from build123d import *

# Parameters (mm, degrees)
SKETCH1_W           = 7
SKETCH1_H           = 7
BOSS_EXTRUDE1_DEPTH = 3
CUT_EXTRUDE1_DEPTH  = 7
CUT_EXTRUDE2_DEPTH  = 11
SKETCH4_R           = 1.8
CUT_EXTRUDE3_DEPTH  = 0.8
CUT_EXTRUDE4_DEPTH  = 0.4


with BuildPart() as part:
    # Sketch1 → Boss-Extrude1 (new body)
    with BuildSketch(Plane(origin=(0, 0, 0), x_dir=(1, 0, 0), z_dir=(0, 1, 0))):
        with Locations((3.5, 3.5)):
            Rectangle(SKETCH1_W, SKETCH1_H)
    extrude(amount=BOSS_EXTRUDE1_DEPTH)

    # Sketch2 → Cut-Extrude1 (cut)
    with BuildSketch(Plane.XY):
        Polygon((0, 0), (0.7, 3), (0, 3), align=None)
        Polygon((7, 0), (6.3, 3), (7, 3), align=None)
    extrude(amount=-CUT_EXTRUDE1_DEPTH, mode=Mode.SUBTRACT)

    # Sketch3 → Cut-Extrude2 (cut)
    with BuildSketch(Plane(origin=(0, 0, 0), x_dir=(0, 0, -1), z_dir=(1, 0, 0))):
        Polygon((0, 0), (0.7, 3), (0, 3), align=None)
        Polygon((7, 3), (6.3, 3), (7, 0), align=None)
    extrude(amount=CUT_EXTRUDE2_DEPTH, mode=Mode.SUBTRACT)

    # Sketch4 → Cut-Extrude3 (cut)
    with BuildSketch(Plane.XZ):
        with Locations(Location((3.5, -3.5, 0), (0, 0, 270))):
            Circle(SKETCH4_R)
    extrude(amount=-CUT_EXTRUDE3_DEPTH, mode=Mode.SUBTRACT)

    # Sketch5 → Cut-Extrude4 (cut)
    with BuildSketch(Plane(origin=(0, 3, 0), x_dir=(1, 0, 0), z_dir=(0, 1, 0))):
        with BuildLine():
            Line((2.030546131, 1.772776287), (2.030546131, 5.272776287))
            Line((2.030546131, 5.272776287), (3.499396292, 5.272776287))
            add(Edge.make_bspline(
                [(3.499396292, 5.272776287), (3.5440361, 5.272501173), (3.63006518, 5.271970977), (3.754480014, 5.268104688), (3.869218418, 5.260004585), (3.974789374, 5.250831153), (4.070685816, 5.2374844), (4.157286901, 5.221495121), (4.23444683, 5.202965752), (4.303291413, 5.180773827), (4.366063686, 5.155374398), (4.424539139, 5.125141932), (4.479360726, 5.089720882), (4.531370453, 5.050332114), (4.580788559, 5.006915106), (4.626260263, 4.958320831), (4.668577803, 4.90527287), (4.707707034, 4.848212589), (4.742177437, 4.787391941), (4.773674335, 4.724764195), (4.799313998, 4.659662899), (4.820492127, 4.592394727), (4.837409543, 4.523105729), (4.849151659, 4.451619746), (4.856482135, 4.378066169), (4.857136528, 4.328382861), (4.857469208, 4.303124845)],
                knots=[0, 0, 0, 0, 1.675828044, 3.229627355, 4.67171229, 5.993455049, 7.206927059, 8.304770529, 9.29850117, 10.183580433, 11.017754134, 11.837875825, 12.650738409, 13.464925643, 14.285328857, 15.117007378, 15.959673368, 16.830859064, 17.711229498, 18.58228265, 19.460420693, 20.334473227, 21.228207035, 22.135446768, 23.052097822, 24, 24, 24, 24], degree=3))
            add(Edge.make_bspline(
                [(4.857469208, 4.303124845), (4.856852136, 4.271306813), (4.855646207, 4.20912561), (4.844548611, 4.117987318), (4.828065847, 4.030911185), (4.804569794, 3.947776576), (4.772263199, 3.869561272), (4.734759192, 3.795169587), (4.690029362, 3.724853862), (4.638377601, 3.659311167), (4.579850151, 3.598483484), (4.51419052, 3.543622601), (4.441867499, 3.494514108), (4.362443578, 3.451441194), (4.276471789, 3.414618521), (4.18357933, 3.383637045), (4.084186726, 3.358421575), (4.015049286, 3.346556943), (3.979664721, 3.34048462)],
                knots=[0, 0, 0, 0, 1.05911256, 2.069797862, 3.05271628, 4.008392045, 4.940519534, 5.866323021, 6.779546087, 7.71056835, 8.640711998, 9.585328432, 10.554502533, 11.547017206, 12.589327225, 13.664782803, 14.804835066, 16, 16, 16, 16], degree=3))
            add(Edge.make_bspline(
                [(3.979664721, 3.34048462), (4.013885569, 3.317819831), (4.080860431, 3.27346175), (4.173524973, 3.200403435), (4.256715746, 3.123723082), (4.319703603, 3.055534143), (4.368103279, 2.995569296), (4.407073288, 2.943123463), (4.44910869, 2.882765916), (4.493797209, 2.814463953), (4.542459952, 2.738821883), (4.593287063, 2.65468189), (4.647342172, 2.562864685), (4.683685664, 2.49872572), (4.702521292, 2.46548462)],
                knots=[0, 0, 0, 0, 1.285445069, 2.515791127, 3.691898215, 4.826622834, 5.420063933, 6.105349801, 6.873086501, 7.723915395, 8.66222816, 9.690593598, 10.803111229, 12, 12, 12, 12], degree=3))
            Line((4.702521292, 2.46548462), (5.126699978, 1.772776287))
            Line((5.126699978, 1.772776287), (4.340041324, 1.772776287))
            Line((4.340041324, 1.772776287), (3.842244849, 2.56714728))
            add(Edge.make_bspline(
                [(3.842244849, 2.56714728), (3.819383068, 2.598961265), (3.775735226, 2.659700703), (3.71272687, 2.746013416), (3.655079817, 2.822847232), (3.604328246, 2.891315046), (3.55790415, 2.949475634), (3.517217149, 2.998342534), (3.483095985, 3.038964357), (3.444487802, 3.079242648), (3.399571281, 3.120637513), (3.343968216, 3.16077219), (3.286869026, 3.192767131), (3.225691806, 3.217180023), (3.154942198, 3.234202313), (3.069889966, 3.245047676), (2.967860868, 3.253049263), (2.894114271, 3.253371714), (2.85436424, 3.253545518)],
                knots=[0, 0, 0, 0, 1.465447777, 2.797841088, 3.997266218, 5.05856206, 5.985598736, 6.780315439, 7.437430484, 7.969193402, 8.866571936, 9.718200644, 10.52825214, 11.309096006, 12.174169268, 13.242355782, 14.513606761, 16, 16, 16, 16], degree=3))
            Line((2.85436424, 3.253545518), (2.703623054, 3.253545518))
            Line((2.703623054, 3.253545518), (2.703623054, 1.772776287))
            Line((2.703623054, 1.772776287), (2.030546131, 1.772776287))
        make_face()
        with BuildLine():
            Line((2.703623054, 3.836878851), (3.245590202, 3.836878851))
            add(Edge.make_bspline(
                [(3.245590202, 3.836878851), (3.287425822, 3.836968507), (3.367129748, 3.837139318), (3.480470316, 3.839613437), (3.581721608, 3.841713365), (3.670277711, 3.846989524), (3.746534832, 3.852218694), (3.810187065, 3.859014719), (3.861770698, 3.867047401), (3.913294077, 3.879536112), (3.966071524, 3.901295225), (4.022322296, 3.932286607), (4.070398439, 3.972490835), (4.112043483, 4.018970988), (4.143812817, 4.073612635), (4.16869572, 4.133981429), (4.181311879, 4.201418818), (4.183343969, 4.24816171), (4.184392285, 4.272275486)],
                knots=[0, 0, 0, 0, 1.697953026, 3.23488743, 4.60134403, 5.807846676, 6.835100678, 7.703488618, 8.405232423, 8.952775585, 9.851109663, 10.713519226, 11.549115941, 12.382556273, 13.233359028, 14.101746968, 15.020727134, 16, 16, 16, 16], degree=3))
            add(Edge.make_bspline(
                [(4.184392285, 4.272275486), (4.183200022, 4.299251728), (4.180899743, 4.351298039), (4.162759412, 4.425360435), (4.131096203, 4.490784365), (4.0876106, 4.547677846), (4.033021276, 4.595719522), (3.967999354, 4.633854155), (3.893027901, 4.662255248), (3.838953649, 4.672743717), (3.810694369, 4.678225005)],
                knots=[0, 0, 0, 0, 1.062977961, 2.050844577, 2.982300261, 3.90936959, 4.856017476, 5.831122378, 6.86654153, 8, 8, 8, 8], degree=3))
            add(Edge.make_bspline(
                [(3.810694369, 4.678225005), (3.801353235, 4.679251395), (3.779212787, 4.681684154), (3.74011538, 4.683246609), (3.690124331, 4.685648271), (3.628634545, 4.686629777), (3.556195371, 4.688350271), (3.472518757, 4.688666197), (3.377870551, 4.689675558), (3.311028641, 4.689523327), (3.275738439, 4.689442953)],
                knots=[0, 0, 0, 0, 0.42127143, 0.998501726, 1.753681744, 2.66564073, 3.755712164, 5.002818897, 6.417592707, 8, 8, 8, 8], degree=3))
            Line((3.275738439, 4.689442953), (2.703623054, 4.689442953))
            Line((2.703623054, 4.689442953), (2.703623054, 3.836878851))
        make_face(mode=Mode.SUBTRACT)
    extrude(amount=-CUT_EXTRUDE4_DEPTH, mode=Mode.SUBTRACT)


solid = part.part
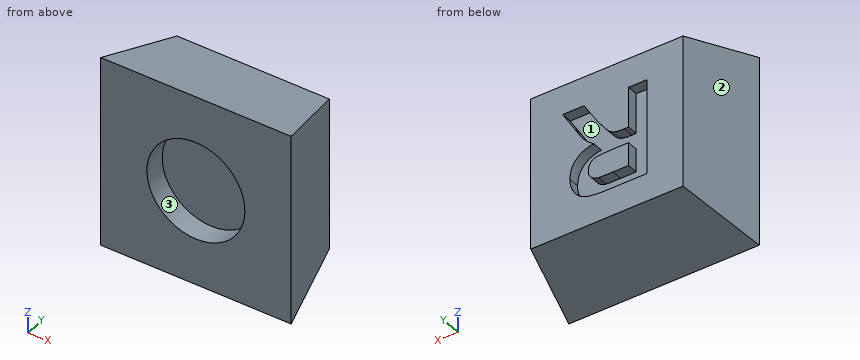
Can you work these out from the model? Positions are in its coordinate system, mm. Face numbers are marked on the shaded views. A direction names the side the tool comes from. Give positions to 0.01 mm unless a question says otherwise; leave off trailing zeros. Write each loop counter-clockwise with the first axis right and the second up, starting at its lowest first coordinate (ties: lowest second). Pieces come first, ordered by that corner, then holes. Notation, with made-up numbers: M 36,27 L 90,27 A16 ccw 90,32 Z; hole C -35,47 d5. An arc over 180 degrees is marked long. Answer in a Markdown table with one row per item. Add a question column.
Item 1: Imagine slicing it at B-B, the plane z = -1.25. Write out the boundary of the cut face in (x, y), plus the area to 3 significant figures.
Item 2: For pin 1 Ø1.5 at (x, y) = (2.5, 0.5) entering from -Z, with a flat end and sliding along its axis, tell me the tip position at first contact or that it passes through.
Item 3: On a 3-axis mill with a long thin cutter (end or side, diameter ignored), from which of +Z, -Z, +X, -X, +Y, -Y can I reach the whole of each face in a straight line? I mean the marked faces 1, 2 and 3. Say none if no direction works.
Item 4: Imagine slicing it at C-C, the plane y = 2.4. Write out the boundary of the cut face in (x, z).
Item 5: Imagine slicing it at A-A, the plane y = 0.55. Write out the boundary of the cut face in (x, z).
Item 6: Please list where these lines run through material, in increasing order: L1, parallel to X at y = 0.4, z = -3.5; L2, parallel to X at y = 2.7, z = -5; L3, parallel to Z at x = 3.75, y = 2.85 (3 decimals).
Evaluation:
| question | item | result |
|---|---|---|
| 1 | outline | M 0,0 L 7,0 L 6.3,3 L 0.7,3 Z |
| 1 | area | 18.9 mm² |
| 2 | pin 1 | stops at z = -7 |
| 3 | face 1 | +Y |
| 3 | face 2 | +Z, -Z, -X, +Y |
| 3 | face 3 | -Y |
| 4 | outline | M 0.56,-6.44 L 6.44,-6.44 L 6.44,-0.56 L 0.56,-0.56 Z |
| 5 | outline | M 0.13,-6.87 L 6.87,-6.87 L 6.87,-0.13 L 0.13,-0.13 Z; hole C 3.5,-3.5 d3.6 |
| 6 | L1 | x = 0.09 to 1.7, 5.3 to 6.91 |
| 6 | L2 | x = 0.63 to 2.03, 4.59 to 6.37 |
| 6 | L3 | z = -6.335 to -5.268, -4.683 to -3.853, -2.695 to -0.665 |
